The figure shows three views and two pictorial views of one solid part (mm, origin at its lowest corner). Answer the questions. A direction names the side the tool comes from. Coordinates: 2 decimals unless noted, no trailing zeros. Loops run counter-clockwise (first coordinate to the right, second up) from the corner with the lowest first, then second, coordinate; pieces in that order, holes last. Notation, with made-up numbers: (-25.5, 35.5) -> (10.5, 35.5) arc R31 ccw to (10.5, 73.5) -> close; hole circle Ø7 at (-35.5, 18). An arc over 180 degrees is marked (long way). Use a Markdown table: item, result. Add a question column.
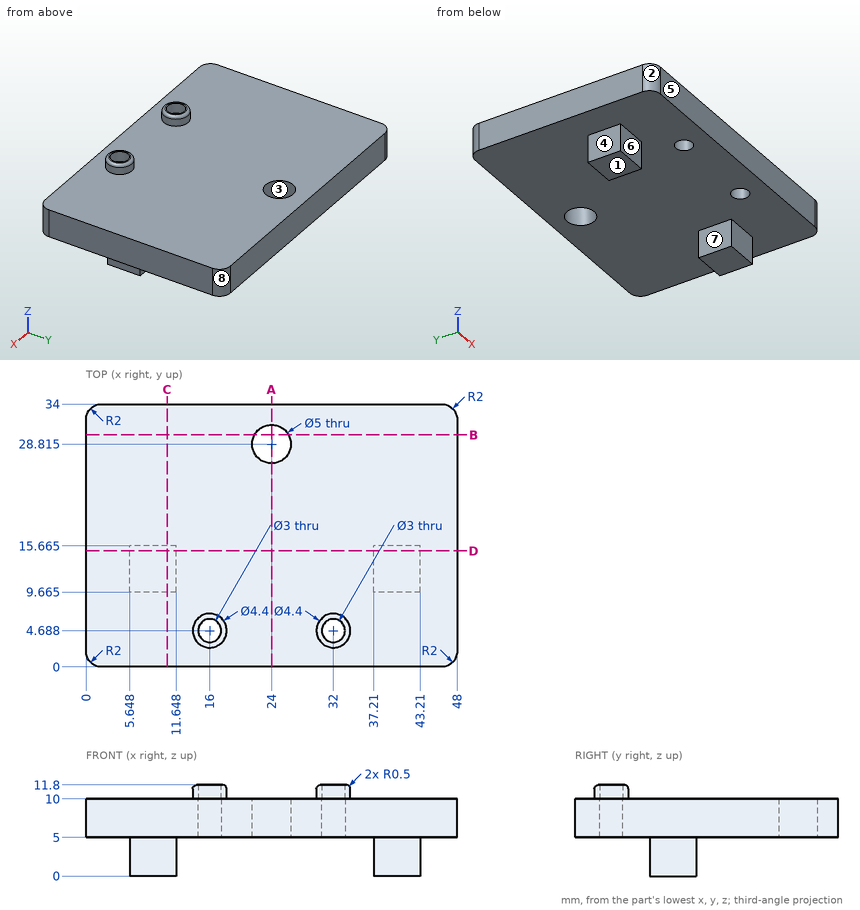
Item 1: Find the intervals of material crossed by probe 1 along Y at (x, z) = (24, 6.2) (1 decimal); probe 2 along X at (y, z) = (11, 1.75); probe 3 along Z at (x, y) = (27, 12.5), in increasing order.
Item 2: For a pull along X with two mould halves and no side action, classify the marked faces 1, 2 and 3 as +X half, -X half, draft (parallel to the pull), parting line (faces both ways), or undercut.
Item 3: Section D-D (y = 15) is taken. Determine the outline of the cut face in (x, z).
Item 4: For the marked faces 4, 5, 6, 7 and 8, determine the directions among +Z, -Z, +X, -X, +Y, -Y from which every point of the face is accessible in a straight line to the end or side of a thin tool.
Item 5: Section B-B (y = 30) is taken. Determine the outline of the cut face in (x, z).
Item 6: Section C-C (x = 10.5) is taken. Determine the outline of the cut face in (y, z) (1 decimal), then the cut area to 3 significant figures.
Item 7: Section A-A (x = 24) is taken. Determine the outline of the cut face in (y, z) (1 decimal), then the cut area to 3 significant figures.
Item 8: Given pin 1 (1.5 mm diameter, centred on y = 12.5, z = 2.5, fed in from -X); pin 2 (5.5 mm diameter, centred on y = 11.5, z = 3, fed in from -X); pin 3 (3.5 mm diameter, centred on x = 16, y = 4.69, fed in from -Z); pin 4 (1.5 mm diameter, centred on x = 9.5, z = 1.5, fed in from -Y) (1 decimal), each flat-ended and moving along its own axis, determine where each tip first touches the part or whether it passes through.
Output:
| question | item | result |
|---|---|---|
| 1 | probe 1 | y = 0 to 26.3, 31.3 to 34 |
| 1 | probe 2 | x = 5.65 to 11.65, 37.21 to 43.21 |
| 1 | probe 3 | z = 5 to 10 |
| 2 | face 1 | draft |
| 2 | face 2 | -X half |
| 2 | face 3 | undercut |
| 3 | outline | (0, 5) -> (5.65, 5) -> (5.65, 0) -> (11.65, 0) -> (11.65, 5) -> (37.21, 5) -> (37.21, 0) -> (43.21, 0) -> (43.21, 5) -> (48, 5) -> (48, 10) -> (0, 10) -> close |
| 4 | face 4 | -Z, -X, +Y, -Y |
| 4 | face 5 | +Z, -Z, +X, -X, -Y |
| 4 | face 6 | -Z, +X, -X, -Y |
| 4 | face 7 | -Z, +Y, -Y |
| 4 | face 8 | +Z, -Z, +X, +Y |
| 5 | outline | (0, 5) -> (21.8, 5) -> (21.8, 10) -> (0, 10) -> close; (26.2, 5) -> (48, 5) -> (48, 10) -> (26.2, 10) -> close |
| 6 | outline | (0, 5) -> (9.7, 5) -> (9.7, 0) -> (15.7, 0) -> (15.7, 5) -> (34, 5) -> (34, 10) -> (0, 10) -> close |
| 6 | area | 200 mm2 |
| 7 | outline | (0, 5) -> (26.3, 5) -> (26.3, 10) -> (0, 10) -> close; (31.3, 5) -> (34, 5) -> (34, 10) -> (31.3, 10) -> close |
| 7 | area | 145 mm2 |
| 8 | pin 1 | stops at x = 5.65 |
| 8 | pin 2 | stops at x = 0 |
| 8 | pin 3 | stops at z = 5 |
| 8 | pin 4 | stops at y = 9.7 |
